```python
from build123d import *

# Parameters (mm, degrees)
SKETCH1_R           = 2.1
BOSS_EXTRUDE1_DEPTH = 3
SKETCH2_W           = 16
SKETCH2_H           = 16.85
BOSS_EXTRUDE2_DEPTH = 3
SKETCH4_W           = 5.55
SKETCH4_H           = 1
BOSS_EXTRUDE3_DEPTH = 3
CHAMFER1_SIZE       = 1
SKETCH3_R           = 3.05
CUT_EXTRUDE1_DEPTH  = 4
FILLET1_R           = 2


with BuildPart() as part:
    # Sketch1 → Boss-Extrude1 (new body)
    with BuildSketch(Plane.XY):
        Polygon((-5.2, 77.75), (7, 77.75), (24.95, 77.75), (24.95, 57.85), (7, 57.85), (7, 52.9), (-5.2, 52.9), align=None)
        with Locations((0.9, 59)):
            Circle(SKETCH1_R, mode=Mode.SUBTRACT)
    extrude(amount=BOSS_EXTRUDE1_DEPTH)

    # Sketch2 → Boss-Extrude2 (add)
    with BuildSketch(Plane(origin=(-52.8, 77.75, 0), x_dir=(0, 0, -1), z_dir=(0, -1, 0))):
        with Locations((5, 69.325)):
            Rectangle(SKETCH2_W, SKETCH2_H)
    extrude(amount=BOSS_EXTRUDE2_DEPTH)

    # Sketch4 → Boss-Extrude3 (add)
    with BuildSketch(Plane(origin=(0, 0, 0), x_dir=(-1, 0, 0), z_dir=(0, 0, -1))):
        with Locations((-19.175, 58.35)):
            Rectangle(SKETCH4_W, SKETCH4_H)
    extrude(amount=BOSS_EXTRUDE3_DEPTH)

    # Chamfer1
    chamfer1_edges = [part.edges().sort_by_distance(p)[0] for p in [
        (7, 57.85, 1.5),
        (16.525, 74.75, 0),
        (19.175, 58.85, 0),
    ]]
    chamfer(chamfer1_edges, length=CHAMFER1_SIZE)

    # Sketch3 → Cut-Extrude1 (cut, through all)
    with BuildSketch(Plane(origin=(0, 74.75, 0), x_dir=(0, 0, -1), z_dir=(0, -1, 0))):
        with Locations((7, 16.525)):
            Circle(SKETCH3_R)
    extrude(amount=-CUT_EXTRUDE1_DEPTH, mode=Mode.SUBTRACT)

    # Fillet1
    fillet1_edges = [part.edges().sort_by_distance(p)[0] for p in [
        (-5.2, 77.75, 1.5),
        (24.95, 57.85, 1.5),
        (7, 52.9, 1.5),
        (-5.2, 52.9, 1.5),
        (24.95, 76.25, -13),
        (8.1, 76.25, -13),
    ]]
    fillet(fillet1_edges, radius=FILLET1_R)


solid = part.part
```
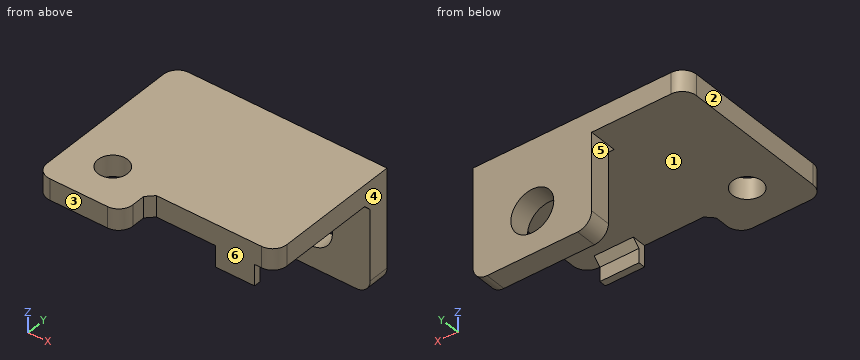
Geometry: final body of the model. Coordinates: model frame, mm. Face numbers are marked on the shaded views. A direction names the side the tool comes from. Give positions to 0.01 mm unless a question says otherwise; leave off trailing zeros. Order: outer loops, then holes, each group sorted by start corner. A loop starts at its lowest first (then second) coordinate and runs counter-clockwise, first axis right, second up. Notation, with made-up numbers: M 68.25,87.25 L 87.25,87.25 A31 cw 87.25,120.25 Z; hole C 51,-12 d8. An arc over 180 degrees is marked long. Answer as CSV lines item,"result". Start each with the question number.
1) Cut plane C-C (x = 20). Output: boundary loops of the cut face in (y, z), then the cut area to 3 significant figures.
2) Cut plane D-D (x = 15). Output: boundary loops of the cut face in (y, z).
3) Cut plane B-B (y = 57.5). Output: boundary loops of the cut face in (x, z), then the cut area to 3 significant figures.
4) Cut plane A-A (z = -7). Output: boundary loops of the cut face in (x, y) (3 decimals).
5) First-contact query: P1, Ø2, axis at y = 75, z = -4, coming from the -X side; P2, Ø4, axis at x = 4.5, z = -5.5, coming from the +Y side; P3, Ø5, axis at x = 20.5, y = 72, coming from the -Z side; P4, Ø10, axis at x = 16.5, y = 58, coming from the -Z side. Flat tips, straight axial feed; report the tip coordinate or a pass-through.
6) Set-up query: the marked faces 4, 5 and 6. Return all of +Z, -Z, +X, -X, +Y, -Y with unobstructed straight access to the full face (end or side cutting, diameter ignored); none if empty.
7) Mould query, pull axis Y, two halves, no side actions, for the marked faces 1, 2 and 3. Classes: +Y half, -Y half, draft (parallel to the pull), parting line (faces both ways), or undercut.
8) Line query: line 1 (Y direction, x = 0.9, z = 1.75); line 2 (Y direction, x = 18, z = -2.5); line 3 (X direction, y = 77.15, z = -7) (3 decimals). Output: solid intervals per line, ascending. Write a range as from..to.
Findings below:
1,outline,"M 57.85,-3 L 58.85,-3 L 58.85,-1 L 59.85,0 L 73.75,0 L 74.75,-1 L 74.75,-13 L 77.75,-13 L 77.75,3 L 57.85,3 Z"
1,area,"103 mm²"
2,outline,"M 57.85,0 L 73.75,0 L 74.75,-1 L 74.75,-4.36 L 77.75,-4.36 L 77.75,3 L 57.85,3 Z; M 74.75,-13 L 77.75,-13 L 77.75,-9.64 L 74.75,-9.64 Z"
3,outline,"M -5.2,0 L -0.57,0 L -0.57,3 L -5.2,3 Z; M 2.37,0 L 7.65,0 L 7.65,3 L 2.37,3 Z"
3,area,"29.7 mm²"
4,outline,"M 8.1,74.75 L 13.475,74.75 L 13.475,77.75 L 8.1,77.75 Z; M 19.575,74.75 L 24.95,74.75 L 24.95,77.75 L 19.575,77.75 Z"
5,P1,"stops at x = 8.1"
5,P2,"passes through"
5,P3,"stops at z = -0.75"
5,P4,"stops at z = -3"
6,face 4,"+Z, -Z, +X, +Y, -Y"
6,face 5,"-Z, -X, +Y, -Y"
6,face 6,"+Z, -Z, +X, -Y"
7,face 1,"undercut"
7,face 2,"draft"
7,face 3,"-Y half"
8,line 1,"y = 52.9..56.9, 61.1..77.75"
8,line 2,"y = 57.85..58.85, 74.75..77.75"
8,line 3,"x = 8.1..13.475, 19.575..24.95"
